Work out the finished part from the listing and answer in its coordinate system (mm). Face numbers are marked on the shaded views. A direction names the side the tool comes from. Round coordinates to 2 decimals unless told otherwise and drop trailing zeros. Loops run counter-clockwise (first coordinate to the right, second up) from the corner with the lowest first, then second, coordinate; pieces in that order, holes last.
from build123d import *

# Parameters (mm, degrees)
EXTRUDE_1_DEPTH         = 100
CUT_EXTRUDE_2_DEPTH     = 1610.175588972
CUT_EXTRUDE_7_DEPTH     = 1610.175588972
HOLE_WIZARD_M6_1_REACH  = 1611.176
HOLE_WIZARD_M6_1_BORE_R = 2.5
CUT_EXTRUDE_8_REACH     = 1611.176


with BuildPart() as part:
    # 草图3 → 凸台-拉伸1 (new body)
    with BuildSketch(Plane(origin=(0, 0, 0), x_dir=(1, 0, 0), z_dir=(0, 1, 0))):
        with BuildLine():
            Line((-139.449188396, -1593.911516947), (-122.018039847, -1394.672577328))
            ThreePointArc((-122.018039847, -1394.672577328), (0, -1400), (122.018039847, -1394.672577328))
            Line((122.018039847, -1394.672577328), (139.449188396, -1593.911516947))
            ThreePointArc((139.449188396, -1593.911516947), (0, -1600), (-139.449188396, -1593.911516947))
        make_face()
    extrude(amount=EXTRUDE_1_DEPTH)

    # 草图6 → 切除-拉伸2 (cut, through all)
    with BuildSketch(Plane(origin=(0, 100, 0), x_dir=(1, 0, 0), z_dir=(0, 1, 0))):
        Polygon((-12.5, -1399.944195316), (12.5, -1399.944195316), (12.5, -1449.944195316), (0, -1449.944195316), (-12.5, -1449.944195316), align=None)
    extrude(amount=-CUT_EXTRUDE_2_DEPTH, mode=Mode.SUBTRACT)

    # 草图8 → 切除-旋转1 (revolve, cut)
    with BuildSketch(Plane(origin=(-35, 0, 0), x_dir=(0, 0, -1), z_dir=(1, 0, 0)), mode=Mode.PRIVATE) as cut_revolve_1_sk:
        Polygon((-1525, 100), (-1530, 100), (-1538.682408883, 50.759612349), (-1538.682408883, 0), (-1525, 0), align=None)
    cut_revolve_1 = revolve(cut_revolve_1_sk.sketch.rotate(Axis((-35, 0, 1525), (0, 1, 0)), 180), axis=Axis((-35, 0, 1525), (0, 1, 0)), mode=Mode.SUBTRACT)

    # 镜向1: 切除-旋转1 across plane
    add(cut_revolve_1.mirror(Plane.ZY), mode=Mode.SUBTRACT)

    # 草图10 → 切除-拉伸7 (cut, through all)
    with BuildSketch(Plane.XZ):
        with BuildLine():
            Line((-134.219843831, 1534.139835061), (-132.040950263, 1509.234967609))
            ThreePointArc((-132.040950263, 1509.234967609), (-92.488537395, 1512.174219609), (-52.872737504, 1514.077102934))
            Line((-52.872737504, 1514.077102934), (-53.745224922, 1539.061873609))
            ThreePointArc((-53.745224922, 1539.061873609), (-94.014750884, 1537.12758957), (-134.219843831, 1534.139835061))
        make_face()
        with BuildLine():
            Line((53.745224922, 1539.061873609), (52.872737504, 1514.077102934))
            ThreePointArc((52.872737504, 1514.077102934), (92.488537395, 1512.174219609), (132.040950263, 1509.234967609))
            Line((132.040950263, 1509.234967609), (134.219843831, 1534.139835061))
            ThreePointArc((134.219843831, 1534.139835061), (94.014750884, 1537.12758957), (53.745224922, 1539.061873609))
        make_face()
    extrude(amount=-CUT_EXTRUDE_7_DEPTH, mode=Mode.SUBTRACT)

    # M6 螺纹孔的螺纹孔钻头1 bore → M6 螺纹孔的螺纹孔钻头1 (cut, up to next)
    with BuildSketch(Plane(origin=(0, 0, 0), x_dir=(-0.0348994967024942, 0, 0.999390827019096), z_dir=(-0.999390827019096, 0, -0.0348994967024942)), mode=Mode.PRIVATE) as hole_wizard_m6_1_sk1:
        with Locations((1526.5, 40)):
            Circle(HOLE_WIZARD_M6_1_BORE_R)
    hole_wizard_m6_1_tool1 = extrude(hole_wizard_m6_1_sk1.sketch, amount=-HOLE_WIZARD_M6_1_REACH, mode=Mode.PRIVATE) & part.part
    hole_wizard_m6_1 = hole_wizard_m6_1_tool1.solids().sort_by_distance((-53.274082, 40, 1525.570097))[0]
    add(hole_wizard_m6_1, mode=Mode.SUBTRACT)

    # 镜向2: M6 螺纹孔的螺纹孔钻头1 across plane
    add(hole_wizard_m6_1.mirror(Plane.ZY), mode=Mode.SUBTRACT)

    # 草图14 → 切除-拉伸8 (cut, up to next)
    with BuildSketch(Plane.XZ, mode=Mode.PRIVATE) as cut_extrude_8_sk1:
        with BuildLine():
            Line((127.029495055, 1451.953772469), (67.310647375, 1398.380948365))
            ThreePointArc((67.310647375, 1398.380948365), (94.682500787, 1396.794624862), (122.018039847, 1394.672577328))
            Line((122.018039847, 1394.672577328), (127.029495055, 1451.953772469))
        make_face()
    cut_extrude_8_tool1 = extrude(cut_extrude_8_sk1.sketch, amount=-CUT_EXTRUDE_8_REACH, mode=Mode.PRIVATE) & part.part
    # 草图14 → 切除-拉伸8 (cut, up to next)
    with BuildSketch(Plane.XZ, mode=Mode.PRIVATE) as cut_extrude_8_sk2:
        with BuildLine():
            Line((-127.029495055, 1451.953772469), (-122.018039847, 1394.672577328))
            ThreePointArc((-122.018039847, 1394.672577328), (-94.682500787, 1396.794624862), (-67.310647375, 1398.380948365))
            Line((-67.310647375, 1398.380948365), (-127.029495055, 1451.953772469))
        make_face()
    cut_extrude_8_tool2 = extrude(cut_extrude_8_sk2.sketch, amount=-CUT_EXTRUDE_8_REACH, mode=Mode.PRIVATE) & part.part
    add(cut_extrude_8_tool1.solids().sort_by_distance((105.520281, 0, 1415.117528))[0], mode=Mode.SUBTRACT)
    add(cut_extrude_8_tool2.solids().sort_by_distance((-105.520281, 0, 1415.117528))[0], mode=Mode.SUBTRACT)


solid = part.part
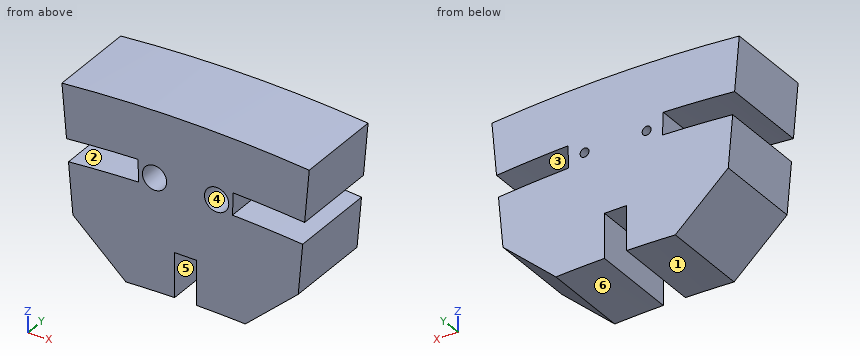
Item 1: Straight lines are drawn through the part: line 1 (X direction, y = 58.5, z = 1532); line 2 (X direction, y = 16.5, z = 1525); line 3 (Z direction, x = -8, y = 62.5). For each, find the intervals that lie inside material, in ascending order.
Item 2: For the marked faces 1, 2 and 3, determine the directions among +Z, -Z, +X, -X, +Y, -Y from which every point of the face is accessible in a straight line to the end or side of a thin tool.
Item 3: Section B-B, the plane z = 1444 is taken. Give the vertices of the cut face in (x, y).
Item 4: Each of these flat-tipped pins is pushed along its axis until it touches: P1, Ø6, axis at y = 74.5, z = 1531.5, coming from the -X side; P2, Ø10, axis at y = 73.5, z = 1434.5, coming from the -X side; P3, Ø10, axis at y = 76, z = 1552.5, coming from the +X side. Where does it stop, or does it pass through?
Item 5: Section D-D, the plane x = 35 is taken. Give the vertices of the cut face in (y, z), plus the area to 3 significant figures.
Item 6: Section C-C, the plane x = 110.5 is taken. Give the vertices of the cut face in (y, z).
Item 7: Section A-A, the plane y = 14 is taken. Give the vertices of the cut face in (x, z).
Item 8: Determine the mould class of the marked faces 4, 5 and 6 for opening direction Z: pulls with the +Z half, pulls with the -Z half, needs draft (parallel to the pull), parting line crosses it, or undercut.
Answer below:
1. line 1: x = -53.5 to -45.14, -24.86 to 24.86, 45.14 to 53.5
1. line 2: x = -53.25 to -48.68, -21.32 to 21.32, 48.68 to 53.25
1. line 3: z = 1449.94 to 1599.98
2. face 1: -Z, +Y, -Y
2. face 2: -X, +Y, -Y
2. face 3: +Y, -Y
3. outline: (-118.16, 0) - (-12.5, 0) - (-12.5, 100) - (-118.16, 100) - close; (12.5, 0) - (118.16, 0) - (118.16, 100) - (12.5, 100) - close
4. P1: stops at x = -134.25
4. P2: stops at x = -113.15
4. P3: stops at x = 136.26
5. outline: (0, 1399.56) - (100, 1399.56) - (100, 1520) - (50.76, 1511.32) - (0, 1511.32) - close; (0, 1538.68) - (50.76, 1538.68) - (100, 1530) - (100, 1599.62) - (0, 1599.62) - close
5. area: 17,700 mm2
6. outline: (0, 1437.13) - (100, 1437.13) - (100, 1510.96) - (0, 1510.96) - close; (0, 1536.03) - (100, 1536.03) - (100, 1596.18) - (0, 1596.18) - close
7. outline: (-139.45, 1593.91) - (-134.22, 1534.14) arc R1540 cw to (-53.75, 1539.06) - (-52.87, 1514.08) arc R1515 ccw to (-132.04, 1509.23) - (-127.03, 1451.95) - (-67.31, 1398.38) arc R1400 cw to (-12.5, 1399.94) - (-12.5, 1449.94) - (12.5, 1449.94) - (12.5, 1399.94) arc R1400 cw to (67.31, 1398.38) - (127.03, 1451.95) - (132.04, 1509.23) arc R1515 ccw to (52.87, 1514.08) - (53.75, 1539.06) arc R1540 cw to (134.22, 1534.14) - (139.45, 1593.91) arc R1600 ccw to start; hole circle Ø27.36 at (-35, 1525); hole circle Ø27.36 at (35, 1525)
8. face 4: undercut
8. face 5: needs draft
8. face 6: pulls with the -Z half
